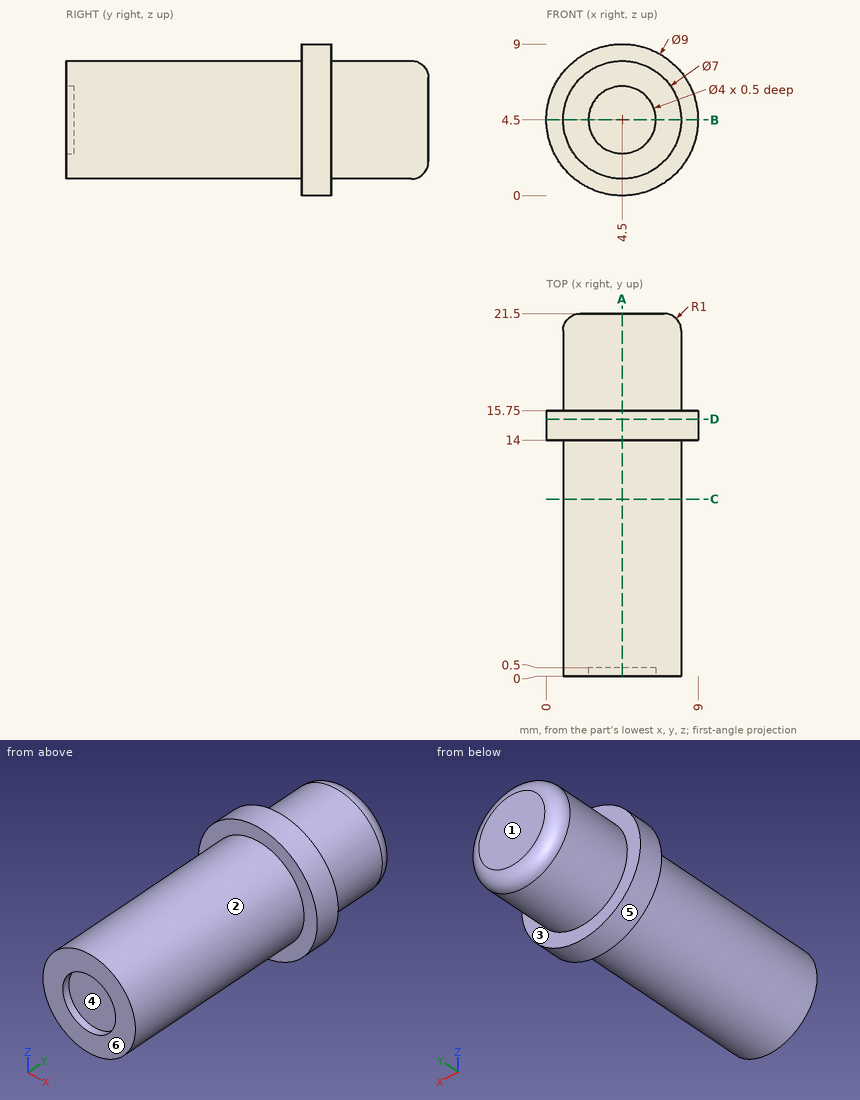
Here's the drawing with two shaded views (mm, measured from the low corner). I have some questions. A direction names the side the tool comes from. Round coordinates to 2 decimals unless told otherwise and drop trailing zeros. Loops run counter-clockwise (first coordinate to the right, second up) from the corner with the lowest first, then second, coordinate; pieces in that order, holes last. Notation, with made-up numbers: M 72.25,-6 L 120.25,-6 A17 cw 120.25,6 Z; hole C 30.5,-14 d11. An arc over 180 degrees is marked long. Answer as CSV lines item,"result".
1) We'd pull the mould along X, two halves only. Please class the marked faces 4, 5 and 6: released by +X, released by -X, zero draft, split by the parting line, or undercut.
From the geometry:
face 4,"undercut"
face 5,"split by the parting line"
face 6,"zero draft"
2) Imagine slicing it at D-D on y = 15.25. List the corners of the cut face in (x, z) for me.
From the geometry:
outline,"C 4.5,4.5 d9"
3) Imagine slicing it at C-C on y = 10.5. List the corners of the cut face in (x, z) for me, and give its area (3 significant figures).
From the geometry:
outline,"C 4.5,4.5 d7"
area,"38.5 mm^2"
4) Imagine slicing it at A-A on x = 4.5. List the corners of the cut face in (y, z) for me.
From the geometry:
outline,"M 0,1 L 14,1 L 14,0 L 15.75,0 L 15.75,1 L 20.5,1 A1 ccw 21.5,2 L 21.5,7 A1 ccw 20.5,8 L 15.75,8 L 15.75,9 L 14,9 L 14,8 L 0,8 L 0,6.5 L 0.5,6.5 L 0.5,2.5 L 0,2.5 Z"
5) For pin 1 Ø3 at (y, z) = (12, 3) entering from -X; pin 2 Ø4 at (x, y) = (5, 9) entering from -Z; pin 3 Ø2 at (x, z) = (4.5, 4.5) entering from -Y, each with a flat end and sliding along its axis, tell me the tip position at first contact or that it passes through.
From the geometry:
pin 1,"x = 1"
pin 2,"z = 1"
pin 3,"y = 0.5"
6) Imagine slicing it at B-B on z = 4.5. List the corners of the cut face in (x, y) for me, and give its area (3 significant figures).
From the geometry:
outline,"M 0,14 L 1,14 L 1,0 L 2.5,0 L 2.5,0.5 L 6.5,0.5 L 6.5,0 L 8,0 L 8,14 L 9,14 L 9,15.75 L 8,15.75 L 8,20.5 A1 ccw 7,21.5 L 2,21.5 A1 ccw 1,20.5 L 1,15.75 L 0,15.75 Z"
area,"152 mm^2"
7) Which directions (+Z, -Z, +X, -X, +Y, -Y) give clear straight access to the entire face, cutting with the end or side of a thin tool? Please do the marked faces 1, 2 and 3.
From the geometry:
face 1,"+Z, -Z, +X, -X, +Y"
face 2,"-Y"
face 3,"+Y"
8) If I drill on probe 1 along X at (y, z) = (0.3, 4.5); probe 2 along Y at (x, z) = (4, 5.75); probe 3 along Y at (x, z) = (3, 1), over which ranges is the centre line in solid material (lowest first)?
From the geometry:
probe 1,"1 to 2.5, 6.5 to 8"
probe 2,"0.5 to 21.5"
probe 3,"14 to 15.75"
